Model file for the job. Use its own axes, mm. Face numbers are marked on the shaded views. A direction names the side the tool comes from. Round coordinates to 2 decimals unless told otherwise and drop trailing zeros. Order: outer loops, then holes, each group sorted by start corner. A loop starts at its lowest first (then second) coordinate and runs counter-clockwise, first axis right, second up. Notation, with made-up numbers: (77.25, 69.25) - (108.25, 69.25) arc R29 ccw to (108.25, 98.25) - close; hole circle Ø11 at (-0.5, -30). An arc over 180 degrees is marked (long way). Use one line per item in the form item = value.
from build123d import *

# Parameters (mm, degrees)
SKETCH1_R                            = 5
SKETCH1_R_2                          = 3
BOSS_EXTRUDE1_DEPTH                  = 1
SKETCH1_3_R                          = 5
SKETCH1_3_R_2                        = 3
BOSS_EXTRUDE2_DEPTH                  = 4
CHAMFER1_SIZE                        = 0.25
SKETCH5_R                            = 5.5
BOSS_EXTRUDE4_DEPTH                  = 4.7625
F_2_0_221_DIAMETER_HOLE1_D           = 5.6134
F_2_0_221_DIAMETER_HOLE1_DEPTH       = 4.265103063
F_2_0_221_DIAMETER_HOLE1_CSINK_D     = 6.8834
F_2_0_221_DIAMETER_HOLE1_CSINK_ANGLE = 90
F_2_0_221_DIAMETER_HOLE1_TIP         = 0.494896937
CHAMFER2_SIZE                        = 0.25
CHAMFER3_SIZE                        = 0.25


with BuildPart() as part:
    # Sketch1 → Boss-Extrude1 (new body)
    # profile 1 of 2: a face of its own
    with BuildSketch(Plane(origin=(0, 0, 0), x_dir=(1, 0, 0), z_dir=(0, 1, 0))):
        with Locations(Location((0, 0, 0), (0, 0, 270))):
            Circle(SKETCH1_R)
        Circle(SKETCH1_R_2, mode=Mode.SUBTRACT)
    # profile 2 of 2: a face of its own
    with BuildSketch(Plane(origin=(0, 0, 0), x_dir=(1, 0, 0), z_dir=(0, 1, 0))):
        Circle(SKETCH1_R_2)
    extrude(amount=BOSS_EXTRUDE1_DEPTH)

    # Sketch1<3> → Boss-Extrude2 (add)
    with BuildSketch(Plane(origin=(0, 0, 0), x_dir=(1, 0, 0), z_dir=(0, 1, 0))):
        with Locations(Location((0, 0, 0), (0, 0, 270))):
            Circle(SKETCH1_3_R)
        with Locations(Location((0, 0, 0), (0, 0, 270))):
            Circle(SKETCH1_3_R_2, mode=Mode.SUBTRACT)
    extrude(amount=BOSS_EXTRUDE2_DEPTH)

    # Chamfer1
    chamfer1_edges = [part.edges().sort_by_distance(p)[0] for p in [
        (0, 1, -3),
        (0, 4, -5),
        (0, 4, -3),
    ]]
    chamfer(chamfer1_edges, length=CHAMFER1_SIZE)

    # Sketch5 → Boss-Extrude4 (add)
    with BuildSketch(Plane(origin=(0, 0, 0), x_dir=(1, 0, 0), z_dir=(0, 1, 0))):
        with Locations(Location((0, 0, 0), (0, 0, 270))):
            Circle(SKETCH5_R)
    extrude(amount=-BOSS_EXTRUDE4_DEPTH)

    # #2 (0.221) Diameter Hole1
    with Locations(Plane(origin=(0, -4.7625, 0), x_dir=(-1, 0, 0), z_dir=(0, -1, 0))):
        with Locations((0, 0)):
            CounterSinkHole(F_2_0_221_DIAMETER_HOLE1_D / 2, F_2_0_221_DIAMETER_HOLE1_CSINK_D / 2, depth=F_2_0_221_DIAMETER_HOLE1_DEPTH, counter_sink_angle=F_2_0_221_DIAMETER_HOLE1_CSINK_ANGLE)
            with Locations((0, 0, -(F_2_0_221_DIAMETER_HOLE1_DEPTH + F_2_0_221_DIAMETER_HOLE1_TIP / 2))):  # 160° drill point
                Cone(0, F_2_0_221_DIAMETER_HOLE1_D / 2, F_2_0_221_DIAMETER_HOLE1_TIP, mode=Mode.SUBTRACT)

    # Chamfer2
    chamfer2_edges = [part.edges().sort_by_distance(p)[0] for p in [
        (0, -4.7625, -5.5),
        (0, 0, -5.5),
    ]]
    chamfer(chamfer2_edges, length=CHAMFER2_SIZE)

    # Chamfer3
    chamfer3_edges = [part.edges().sort_by_distance(p)[0] for p in [
        (0, 0, -5),
    ]]
    chamfer(chamfer3_edges, length=CHAMFER3_SIZE - 0.0001)  # a hair under: the kernel refuses the full size


solid = part.part
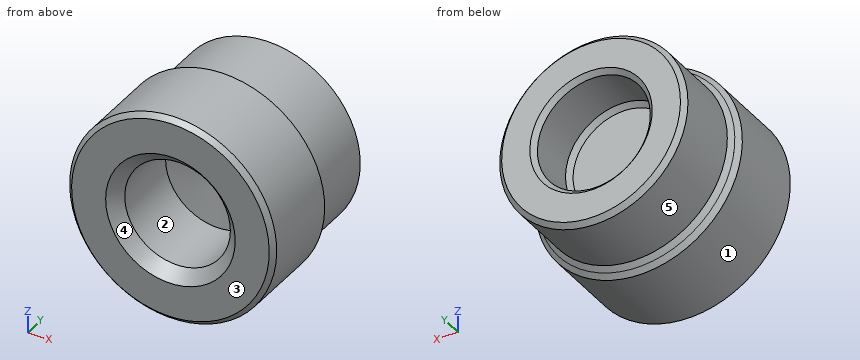
(1) Slice it at A-A on y = -1.25. Give the cut face in (x, z).
Report:
outline = circle Ø11 at (0, 0); hole circle Ø5.61 at (0, 0)
(2) Pull direction X, two halves, no side cores. Call the marked faces 1, 2 and 3: released by +X, released by -X, zero draft, split by the parting line, or undercut.
Report:
face_1 = split by the parting line
face_2 = undercut
face_3 = zero draft
(3) Tool access for the marked faces 4 and 5: list every direction of +Z, -Z, +X, -X, +Y, -Y with a clear straight run to the whole face (end or side of a thin tool).
Report:
face_4 = -Y
face_5 = +Y
(4) Pin check, flat tips, straight feed: pin 1 (1 mm diameter, centred on x = 0.5, z = -2, fed in from -Y); pin 2 (2 mm diameter, centred on y = 2.5, z = 3, fed in from +X); pin 3 (1 mm diameter, centred on x = 2, y = 1.5, fed in from +Z). Stop position of each tip, or through.
Report:
pin_1 = -0.45
pin_2 = 4.58
pin_3 = 4.77
(5) Slice it at B-B on y = 1.5. Give the cut face in (x, z), then the cut area to 3 significant figures.
Report:
outline = circle Ø10 at (0, 0); hole circle Ø6 at (0, 0)
area = 50.3 mm2
(6) Probe probe 1 along X at (y, z) = (2.95, 0); probe 2 along X at (y, z) = (-1.5, 1); probe 3 along Z at (x, y) = (2.5, -4.25). List the from-to ranges inside material, lowest first. Write a range as [from, to].
Report:
probe_1 = [-5, -3], [3, 5]
probe_2 = [-5.41, -2.62], [2.62, 5.41]
probe_3 = [-4.9, -1.53], [1.53, 4.9]
